```python
from build123d import *

# Parameters (mm, degrees)
F0_R     = 26.2509
F3_DEPTH = 457.2
F4_DEPTH = 1066.8


with BuildPart() as f2:
    # F2: sweep along a path in F1
    with BuildLine(Plane.XZ) as f2_path:
        ThreePointArc((0, 0), (27.8387939753, -11.5312060247), (39.37, -39.37))
    # F0 (on Right) → F2 (sweep)
    with BuildSketch(Plane.YZ):
        Circle(F0_R)
    sweep(path=f2_path.line)

    # F3 (add): a face of the model
    f3_faces = [f2.faces().sort_by_distance(p)[0] for p in [
        (0, 0, 0),
    ]]
    extrude(f3_faces, amount=F3_DEPTH)

    # F4 (add): a face of the model
    f4_faces = [f2.faces().sort_by_distance(p)[0] for p in [
        (39.37, 0, -39.37),
    ]]
    extrude(f4_faces, amount=F4_DEPTH)


solid = f2.part
```
For this review, take the finished solid that the model builds, in its own axes (mm). A direction names the side the tool comes from. Round coordinates to 2 decimals unless told otherwise and drop trailing zeros. Write each loop counter-clockwise with the first axis right and the second up, starting at its lowest first coordinate (ties: lowest second). Pieces come first, ordered by that corner, then holes. Notation, with made-up numbers: (85.5, 32.5) - (95.5, 32.5) arc R13 ccw to (95.5, 54.5) - close; hole circle Ø10 at (3.25, 80). An arc over 180 degrees is marked (long way). Answer as a JSON object with one key per item and string values.
1. We need section B-B on x = -71.5. Give the boundary of the cut face in (y, z), then the cut area to 3 significant figures.
Response values:
{"outline": "circle Ø52.5 at (0, 0)", "area": "2,160 mm2"}
2. For pin 1 Ø6 at (x, y) = (-111, 20.5) entering from -Z; pin 2 Ø8 at (y, z) = (-5.5, -563) entering from +X; pin 3 Ø2 at (x, y) = (-229, 1) entering from -Z, all flat-tipped, find the tip position at first contact; note any pin that passes through.
Response values:
{"pin 1": "stops at z = -19.57", "pin 2": "stops at x = 65.58", "pin 3": "stops at z = -26.25"}
3. To check wall thickness, follow line 1 along X through (y, z) = (2, -758); line 2 along X through (y, z) = (-0.5, -811.5); line 3 along Z through (x, y) = (-419, 3). State the ranges of each line that lie inside material, in increasing order.
Response values:
{"line 1": "x = 13.2 to 65.54", "line 2": "x = 13.12 to 65.62", "line 3": "z = -26.08 to 26.08"}
4. We need section A-A on y = 0. Give the boundary of the cut face in (x, z), then the cut area to 3 significant figures.
Response values:
{"outline": "(-457.2, -26.25) - (0, -26.25) arc R13.12 cw to (13.12, -39.37) - (13.12, -1106.17) - (65.62, -1106.17) - (65.62, -39.37) arc R65.62 ccw to (0, 26.25) - (-457.2, 26.25) - close", "area": "83,300 mm2"}
5. Tool access review of faces 1 (the face through (-225.4, -5.691, 25.627)), 2 (the face through (-457.2, 0, 0)), 3 (the face through (31.485, 25.039, -565.302)): name each direction out of +Z, -Z, +X, -X, +Y, -Y from which nothing blocks a thin tool from reaching the whole face with its end or side.
Response values:
{"face 1": "-X", "face 2": "+Z, -Z, -X, +Y, -Y", "face 3": "-Z"}
6. We need section C-C on z = -979. Give the boundary of the cut face in (x, y), then the cut area to 3 significant figures.
Response values:
{"outline": "circle Ø52.5 at (39.37, 0)", "area": "2,160 mm2"}
